The figure shows three views and two pictorial views of one solid part (mm, origin at its lowest corner). Answer the questions. A direction names the side the tool comes from. Coordinates: 2 decimals unless noted, no trailing zeros. Order: outer loops, then holes, each group sorted by start corner. A loop starts at its lowest first (then second) coordinate and runs counter-clockwise, first axis right, second up. Notation, with made-up numbers: (8.5, -16.75) -> (65.5, -16.75) arc R25 ccw to (65.5, 1.25) -> close; hole circle Ø3 at (3.25, 80.25). An arc over 180 degrees is marked (long way). Return JSON: item names as keys, results as strings.
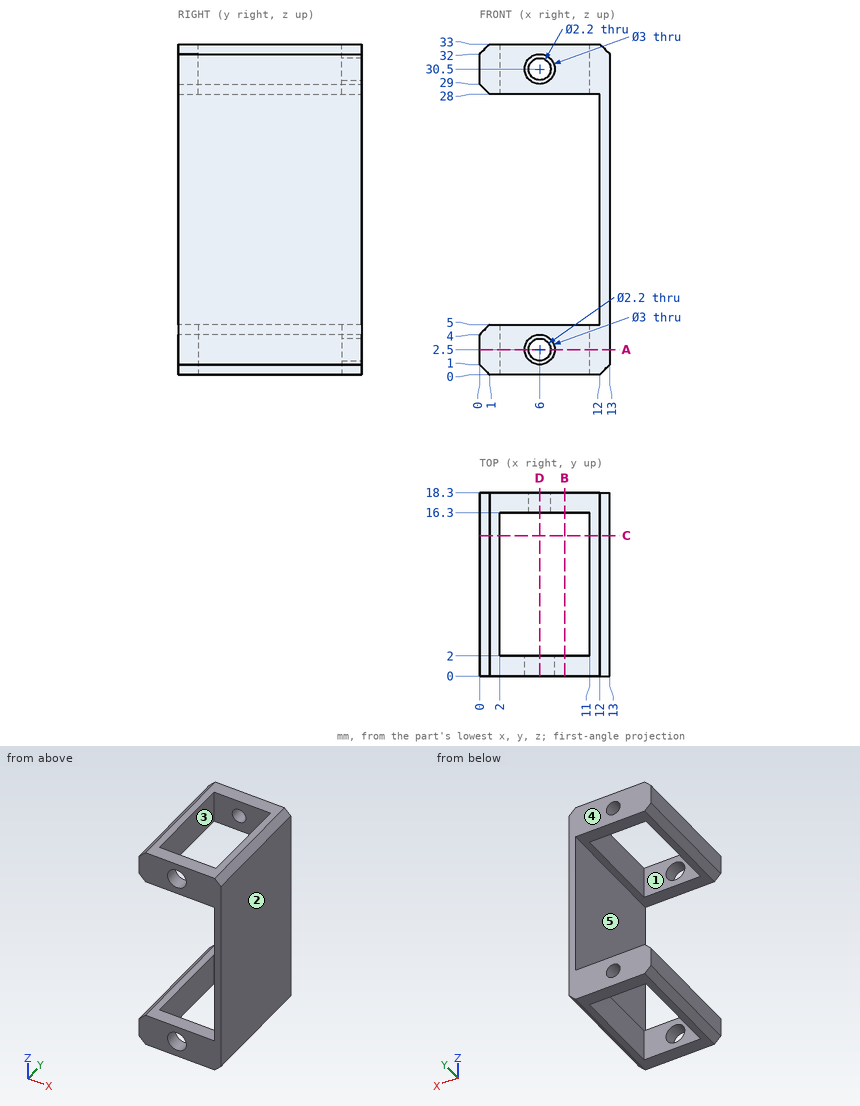
Item 1: Which of the six approach directions +Z, -Z, +X, -X, +Y, -Y give full straight-line access (tool end or side, diameter ignored) to the marked faces 1 and 2?
Answer list:
{"face 1": "+Z, -Z", "face 2": "+Z, -Z, +X, +Y, -Y"}
Item 2: The part is cut by section D-D on x = 6. Count the separate pieces of the cut face and the enclosed holes in it, plus the area to 3 significant figures.
Answer list:
{"separate pieces": "8", "enclosed holes": "0", "area": "19.2 mm2"}
Item 3: A flat-ended cylindrical pin translates along its axis: pin 1 (5.5 mm diameter, centred on y = 6.5, z = 19.5, fed in from -X). Find the tip coordinate at first contact, or state that the pin passes through.
Answer list:
{"pin 1": "x = 12"}
Item 4: The part is cut by section B-B on x = 8.5. Determine the outline of the cut face in (y, z).
Answer list:
{"outline": "(0, 0) -> (2, 0) -> (2, 5) -> (0, 5) -> close; (0, 28) -> (2, 28) -> (2, 33) -> (0, 33) -> close; (16.3, 0) -> (18.3, 0) -> (18.3, 5) -> (16.3, 5) -> close; (16.3, 28) -> (18.3, 28) -> (18.3, 33) -> (16.3, 33) -> close"}
Item 5: The part is cut by section A-A on z = 2.5. Determine the outline of the cut face in (x, y).
Answer list:
{"outline": "(0, 0) -> (4.5, 0) -> (4.5, 2) -> (2, 2) -> (2, 16.3) -> (4.9, 16.3) -> (4.9, 18.3) -> (0, 18.3) -> close; (7.1, 16.3) -> (11, 16.3) -> (11, 2) -> (7.5, 2) -> (7.5, 0) -> (13, 0) -> (13, 18.3) -> (7.1, 18.3) -> close"}
Item 6: Determine the mould class of the marked faces 3, 4 and 5 for opening direction X: pulls with the +X half, pulls with the -X half, needs draft (parallel to the pull), parting line crosses it, or undercut.
Answer list:
{"face 3": "undercut", "face 4": "needs draft", "face 5": "pulls with the -X half"}
Item 7: The part is cut by section C-C on y = 14. Determine the outline of the cut face in (x, z).
Answer list:
{"outline": "(0, 1) -> (1, 0) -> (2, 0) -> (2, 5) -> (1, 5) -> (0, 4) -> close; (0, 29) -> (1, 28) -> (2, 28) -> (2, 33) -> (1, 33) -> (0, 32) -> close; (11, 0) -> (12, 0) -> (13, 1) -> (13, 32) -> (12, 33) -> (11, 33) -> (11, 28) -> (12, 28) -> (12, 5) -> (11, 5) -> close"}
Item 8: Find the intervals of material crossed by probe 1 along X at (y, z) = (3.5, 2); probe 2 along X at (y, z) = (1.3, 2.5); probe 3 along Y at (x, z) = (4.75, 29), in increasing order.
Answer list:
{"probe 1": "0 to 2, 11 to 13", "probe 2": "0 to 4.5, 7.5 to 13", "probe 3": "0 to 2, 16.3 to 18.3"}
